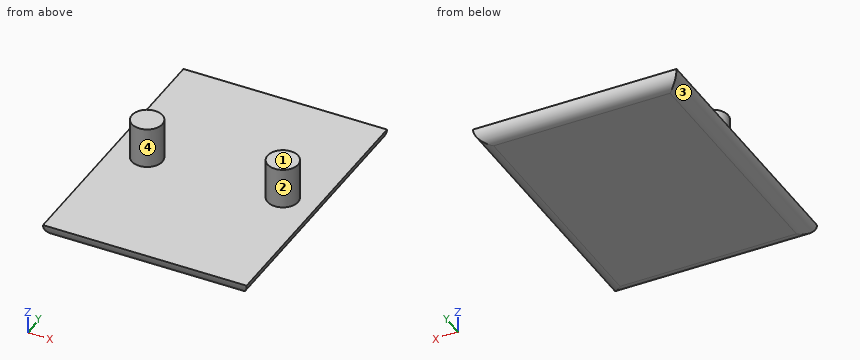
```python
from build123d import *

# Parameters (mm, degrees)
SKETCH1_W           = 30
SKETCH1_H           = 40
SKETCH1_R           = 2.25
BOSS_EXTRUDE1_DEPTH = 2
SKETCH1_4_R         = 2.25
BOSS_EXTRUDE2_DEPTH = 8
FILLET1_R           = 2


with BuildPart() as part:
    # Sketch1 → Boss-Extrude1 (new body)
    with BuildSketch(Plane.XY):
        Rectangle(SKETCH1_W, SKETCH1_H)
        with Locations((-10, 0)):
            Circle(SKETCH1_R, mode=Mode.SUBTRACT)
        with Locations(Location((10, 0, 0), (0, 0, 180))):
            Circle(SKETCH1_R, mode=Mode.SUBTRACT)
    extrude(amount=BOSS_EXTRUDE1_DEPTH)

    # Sketch1<4> → Boss-Extrude2 (add)
    with BuildSketch(Plane.XY):
        with Locations((-10, 0)):
            Circle(SKETCH1_4_R)
        with Locations(Location((10, 0, 0), (0, 0, 180))):
            Circle(SKETCH1_4_R)
    extrude(amount=BOSS_EXTRUDE2_DEPTH)

    # Fillet1
    fillet1_edges = [part.edges().sort_by_distance(p)[0] for p in [
        (0, 20, 0),
        (-15, 0, 0),
        (0, -20, 0),
        (15, 0, 0),
    ]]
    fillet(fillet1_edges, radius=FILLET1_R - 0.0001)  # a hair under: the kernel refuses the full size


solid = part.part
```
Here's how the part is built. I have some questions about the finished solid (model axes, mm). Face numbers are marked on the shaded views. Coordinates: 2 decimals unless noted, no trailing zeros. Loops run counter-clockwise (first coordinate to the right, second up) from the corner with the lowest first, then second, coordinate; pieces in that order, holes last. Notation, with made-up numbers: M 25,-22.75 L 65,-22.75 A30 cw 65,6.25 Z; hole C 23,7.5 d7. An arc over 180 degrees is marked long. One line per item, written item: value.
1. Thinking about a two-plate mould opening in X: for the marked faces 1, 2, 3 and 4, which applies, +X half, -X half, draft (parallel to the pull), parting line (faces both ways), or undercut?
Geometry says:
face 1: draft
face 2: undercut
face 3: -X half
face 4: undercut
2. Will these pins go through, and if not, where does the flat tip stop? pin 1 Ø10 at (x, y) = (2.5, -8.5) entering from +Z; pin 2 Ø2 at (y, z) = (-0.5, 4.5) entering from -X.
Geometry says:
pin 1: stops at z = 2
pin 2: stops at x = -12.25
3. Please list where these lines run through material, in increasing order: probe 1 along Z at (x, y) = (-10.75, 6); probe 2 along X at (y, z) = (1, 7); probe 3 along X at (y, z) = (-0.5, 3.5).
Geometry says:
probe 1: z = 0 to 2
probe 2: x = -12.02 to -7.98, 7.98 to 12.02
probe 3: x = -12.19 to -7.81, 7.81 to 12.19
4. Imagine slicing it at A-A (z = 6.75). List the corners of the cut face in (x, y) for me.
Geometry says:
outline: C -10,0 d4.5; C 10,0 d4.5
